Geometry check sheet. Reference: the model listing, model coordinates, mm. Face numbers are marked on the shaded views. A direction names the side the tool comes from. Coordinates: 2 decimals unless noted, no trailing zeros. Loops run counter-clockwise (first coordinate to the right, second up) from the corner with the lowest first, then second, coordinate; pieces in that order, holes last.
from build123d import *

# Parameters (mm, degrees)
F0_R     = 10
F0_R_2   = 2.5
F1_DEPTH = 25
F2_R     = 5
F2_R_2   = 2.5
F3_DEPTH = 12.5
F5_W     = 4.468582
F5_H     = 22.723214
F6_DEPTH = 5


with BuildPart() as f1:
    # F0 (on Top) → F1 (new body)
    with BuildSketch(Plane.XY):
        Circle(F0_R)
        Circle(F0_R_2, mode=Mode.SUBTRACT)
    extrude(amount=F1_DEPTH)

    # F2 (on face) → F3 (cut)
    with BuildSketch(Plane.XY.offset(25)):
        Circle(F2_R)
        Circle(F2_R_2, mode=Mode.SUBTRACT)
    extrude(amount=-F3_DEPTH, mode=Mode.SUBTRACT)

    # F5 (on offset) → F6 (cut)
    with BuildSketch(Plane.XZ.offset(10)):
        with Locations((6.929936, 12.65571)):
            Rectangle(F5_W, F5_H)
    extrude(amount=-F6_DEPTH, mode=Mode.SUBTRACT)


solid = f1.part
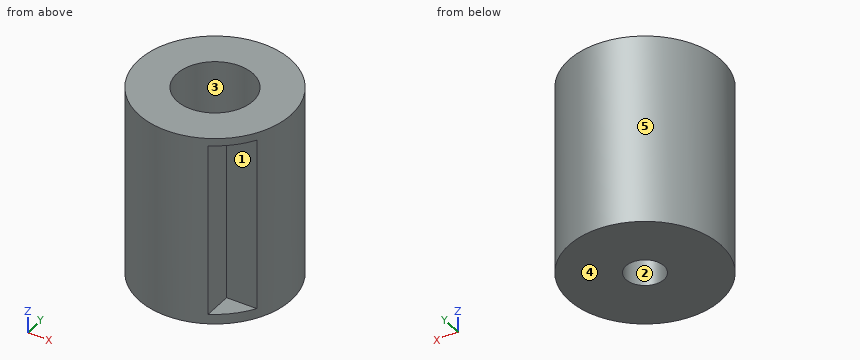
1) Material ranges on probe 1 along Y at (x, z) = (2.75, 18); probe 2 along Z at (x, y) = (4, 2); probe 3 along Y at (x, z) = (3.5, 14.25), recorded low to high.
Data:
probe 1: y = -9.61 to -4.18, 4.18 to 9.61
probe 2: z = 0 to 12.5
probe 3: y = -9.37 to -3.57, 3.57 to 9.37
2) Section check A-A on y = 0. Record the cut outline in (x, z).
Data:
outline: (-10, 0) - (-2.5, 0) - (-2.5, 12.5) - (-5, 12.5) - (-5, 25) - (-10, 25) - close; (2.5, 0) - (10, 0) - (10, 25) - (5, 25) - (5, 12.5) - (2.5, 12.5) - close
3) Mould release check, pull along Y, two halves, no side actions. Record for the marked faces 3, 4 and 5: +Y half, -Y half, draft (parallel to the pull), parting line (faces both ways), or undercut.
Data:
face 3: undercut
face 4: draft
face 5: parting line
4) Section check B-B on z = 14. Record the cut outline in (x, y).
Data:
outline: (4.7, -8.83) - (4.7, -5) - (8.66, -5) arc R10 ccw (long way) to start; hole circle Ø10 at (0, 0)
5) Depth check by flat-ended pin: pin 1 (4 mm diameter, centred on x = 6, z = 11, fed in from +Y); pin 2 (1.2 mm diameter, centred on x = 6.5, z = 8, fed in from -Y); pin 3 (1.5 mm diameter, centred on y = 5, z = 19.5, fed in from +X). Enter the tip coordinate at first touch or a pass-through.
Data:
pin 1: stops at y = 9.17
pin 2: stops at y = -5
pin 3: stops at x = 9.05
6) Section check D-D on y = -6.5. Record the cut outline in (x, z), and give its area (3 significant figures).
Data:
outline: (-7.6, 0) - (7.6, 0) - (7.6, 1.29) - (4.7, 1.29) - (4.7, 24.02) - (7.6, 24.02) - (7.6, 25) - (-7.6, 25) - close
area: 314 mm2
7) Access from +Z, -Z, +X, -X, +Y, -Y to the whole of each face (thin tool, end or side, straight path). Record for the marked faces 1 and 2.
Data:
face 1: +X, -Y
face 2: +Z, -Z
8) Section check C-C on x = 7. Record the cut outline in (y, z), and give its area (3 significant figures).
Data:
outline: (-7.14, 0) - (7.14, 0) - (7.14, 25) - (-7.14, 25) - (-7.14, 24.02) - (-5, 24.02) - (-5, 1.29) - (-7.14, 1.29) - close
area: 308 mm2
